```python
from build123d import *

# Parameters (mm, degrees)
SKETCH3_W           = 70
SKETCH3_H           = 42.5
BOSS_EXTRUDE1_DEPTH = 3
SKETCH4_R           = 10.05
SKETCH4_R_2         = 1.525
BOSS_EXTRUDE2_DEPTH = 3
BOSS_EXTRUDE3_DEPTH = 35
SKETCH6_R           = 3.15
CUT_EXTRUDE1_DEPTH  = 5


with BuildPart() as part:
    # Sketch3 → Boss-Extrude1 (new body)
    with BuildSketch(Plane(origin=(0, 0, 0), x_dir=(1, 0, 0), z_dir=(0, 1, 0))):
        Rectangle(SKETCH3_W, SKETCH3_H)
    extrude(amount=BOSS_EXTRUDE1_DEPTH)

    # Sketch4 → Boss-Extrude2 (add)
    with BuildSketch(Plane.XY.offset(21.25)):
        with BuildLine():
            Line((-35, 3), (-17.290526546, 41.876400939))
            ThreePointArc((-17.290526546, 41.876400939), (0, 53), (17.290526546, 41.876400939))
            Line((17.290526546, 41.876400939), (35, 3))
            Line((35, 3), (-35, 3))
        make_face()
        with Locations((0, 25.25)):
            Circle(SKETCH4_R, mode=Mode.SUBTRACT)
        with Locations((-13.774757254, 25.25)):
            Circle(SKETCH4_R_2, mode=Mode.SUBTRACT)
        with Locations((-12.990381057, 32.75)):
            Circle(SKETCH4_R_2, mode=Mode.SUBTRACT)
        with Locations((12.990381057, 32.75)):
            Circle(SKETCH4_R_2, mode=Mode.SUBTRACT)
        with Locations((6.887378627, 37.179289713)):
            Circle(SKETCH4_R_2, mode=Mode.SUBTRACT)
        with Locations((0, 10.25)):
            Circle(SKETCH4_R_2, mode=Mode.SUBTRACT)
        with Locations((6.887378627, 13.320710287)):
            Circle(SKETCH4_R_2, mode=Mode.SUBTRACT)
    extrude(amount=-BOSS_EXTRUDE2_DEPTH)

    # Sketch5 → Boss-Extrude3 (add)
    with BuildSketch(Plane(origin=(0, 0, 18.25), x_dir=(-1, 0, 0), z_dir=(0, 0, -1))):
        with BuildLine():
            Line((-17.849242405, 13), (-17.849242405, 3))
            Line((-17.849242405, 3), (17.849242405, 3))
            Line((17.849242405, 3), (17.849242405, 13))
            Line((17.849242405, 13), (14.849242405, 13))
            ThreePointArc((14.849242405, 13), (0, 6), (-14.849242405, 13))
            Line((-14.849242405, 13), (-17.849242405, 13))
        make_face()
    extrude(amount=BOSS_EXTRUDE3_DEPTH)

    # Sketch6 → Cut-Extrude1 (cut)
    with BuildSketch(Plane(origin=(0, 3, 0), x_dir=(1, 0, 0), z_dir=(0, 1, 0))):
        with Locations(Location((-26, 12.25, 0), (0, 0, 270))):
            Circle(SKETCH6_R)
        with Locations(Location((26, 12.25, 0), (0, 0, 270))):
            Circle(SKETCH6_R)
        with Locations(Location((26, -12.25, 0), (0, 0, 270))):
            Circle(SKETCH6_R)
        with Locations(Location((-26, -12.25, 0), (0, 0, 270))):
            Circle(SKETCH6_R)
    extrude(amount=-CUT_EXTRUDE1_DEPTH, mode=Mode.SUBTRACT)


solid = part.part
```
CAD build for the part. Positions are in the model's coordinates, mm. A direction names the side the tool comes from. Round coordinates to 2 decimals unless told otherwise and drop trailing zeros. Order: outer loops, then holes, each group sorted by start corner. A loop starts at its lowest first (then second) coordinate and runs counter-clockwise, first axis right, second up. Notation, with made-up numbers: (54, 34) - (83, 34) arc R9 ccw to (83, 51) - close; hole circle Ø8 at (40, 63.5). An arc over 180 degrees is marked (long way). Answer in a Markdown table with one row per item. Add a question column.
(1) Band-saw the part on C-C on x = 26. List the corners of the cut face in (y, z), and give its area (3 significant figures).
(2) Band-saw the part on A-A on z = -12.25. List the corners of the cut face in (x, y).
(3) Drop flat-ended pins along their axis: pin 1 Ø0.9 at (x, z) = (17, -1.5) entering from +Y; pin 2 Ø3 at (y, z) = (7.5, 6) entering from +X; pin 3 Ø3 at (x, y) = (3, 7) entering from -Z. Give the stop position or say it passes through.
(4) Band-saw the part on B-B on y = 32.75. List the corners of the cut face in (x, z).
(5) Band-saw the part on D-D on z = -7.5. List the corners of the cut face in (x, y), and give its area (3 significant figures).
(6) 3-axis set-ups, long thin cutter, end or side, ignore diameter. For faces 4 (the face through (-17.849, 8, 1)), 5 (the face through (0, 6, 1)), 6 (the face through (17.849, 8, 1)): which of +Z, -Z, +X, -X, +Y, -Y reach the whole face in a straight line?
(7) Mould opens along Z. For faces 1 (the face through (0, 15, 21.25)), 2 (the face through (35, 1, 0)), 3 (the face through (-27.917, 1.521, -14.75)) say: +Z half, -Z half, draft (parallel to the pull), parting line (faces both ways), or undercut.
(8) Probe L1, parallel to Y at x = 0, z = 20.25 (3 decimals); L2, parallel to X at y = 2.2, z = 12.25; L3, parallel to Z at x = 10.5, y = 40. List the from-to ranges inside material, lowest first. Write a range as [from, to].
Data:
| question | item | result |
|---|---|---|
| 1 | outline | (0, -21.25) - (3, -21.25) - (3, -15.4) - (0, -15.4) - close; (0, -9.1) - (3, -9.1) - (3, 9.1) - (0, 9.1) - close; (0, 15.4) - (3, 15.4) - (3, 18.25) - (22.76, 18.25) - (22.76, 21.25) - (0, 21.25) - close |
| 1 | area | 149 mm^2 |
| 2 | outline | (-35, 0) - (-29.15, 0) - (-29.15, 3) - (-35, 3) - close; (-22.85, 0) - (22.85, 0) - (22.85, 3) - (17.85, 3) - (17.85, 13) - (14.85, 13) arc R19.25 cw to (-14.85, 13) - (-17.85, 13) - (-17.85, 3) - (-22.85, 3) - close; (29.15, 0) - (35, 0) - (35, 3) - (29.15, 3) - close |
| 3 | pin 1 | stops at y = 13 |
| 3 | pin 2 | stops at x = 17.85 |
| 3 | pin 3 | stops at z = -16.75 |
| 4 | outline | (-21.45, 18.25) - (-14.52, 18.25) - (-14.52, 21.25) - (-21.45, 21.25) - close; (-11.47, 18.25) - (-6.69, 18.25) - (-6.69, 21.25) - (-11.47, 21.25) - close; (6.69, 18.25) - (11.47, 18.25) - (11.47, 21.25) - (6.69, 21.25) - close; (14.52, 18.25) - (21.45, 18.25) - (21.45, 21.25) - (14.52, 21.25) - close |
| 5 | outline | (-35, 0) - (35, 0) - (35, 3) - (17.85, 3) - (17.85, 13) - (14.85, 13) arc R19.25 cw to (-14.85, 13) - (-17.85, 13) - (-17.85, 3) - (-35, 3) - close |
| 5 | area | 422 mm^2 |
| 6 | face 4 | -Z, -X, +Y |
| 6 | face 5 | -Z, +Y |
| 6 | face 6 | -Z, +X, +Y |
| 7 | face 1 | +Z half |
| 7 | face 2 | draft |
| 7 | face 3 | undercut |
| 8 | L1 | y = [0, 8.725], [11.775, 15.2], [35.3, 53] |
| 8 | L2 | x = [-35, -29.15], [-22.85, 22.85], [29.15, 35] |
| 8 | L3 | z = [18.25, 21.25] |
